Design review of the part built by this model. Coordinates are the model's own, in mm. Face numbers are marked on the shaded views. A direction names the side the tool comes from. Give positions to 0.01 mm unless a question says otherwise; leave off trailing zeros. Loops run counter-clockwise (first coordinate to the right, second up) from the corner with the lowest first, then second, coordinate; pieces in that order, holes last.
from build123d import *

# Parameters (mm, degrees)
SKETCH1_W           = 36
SKETCH1_H           = 36
BOSS_EXTRUDE1_DEPTH = 10
SKETCH2_W           = 25
SKETCH2_H           = 25
BOSS_EXTRUDE2_DEPTH = 2.5
SKETCH3_R           = 4
BOSS_EXTRUDE3_DEPTH = 12
SKETCH4_R           = 6.5
BOSS_EXTRUDE4_DEPTH = 5
SKETCH5_R           = 5
CUT_EXTRUDE1_DEPTH  = 3
FILLET1_R           = 4
FILLET2_R           = 4
SKETCH7_R           = 1.5
CUT_EXTRUDE2_DEPTH  = 5
SKETCH8_R           = 1.5
CUT_EXTRUDE3_DEPTH  = 5
FILLET3_R           = 1


with BuildPart() as part:
    # Sketch1 → Boss-Extrude1 (new body)
    with BuildSketch(Plane.XY):
        with Locations((18, 18)):
            Rectangle(SKETCH1_W, SKETCH1_H)
    extrude(amount=BOSS_EXTRUDE1_DEPTH)

    # Sketch2 → Boss-Extrude2 (add)
    with BuildSketch(Plane.XY.offset(10)):
        with Locations((18, 18)):
            Rectangle(SKETCH2_W, SKETCH2_H)
    extrude(amount=BOSS_EXTRUDE2_DEPTH)

    # Sketch3 → Boss-Extrude3 (add)
    with BuildSketch(Plane.XY.offset(12.5)):
        with Locations((18, 18)):
            Circle(SKETCH3_R)
    extrude(amount=BOSS_EXTRUDE3_DEPTH)

    # Sketch4 → Boss-Extrude4 (add)
    with BuildSketch(Plane.XY.offset(24.5)):
        with Locations((18, 18)):
            Circle(SKETCH4_R)
    extrude(amount=BOSS_EXTRUDE4_DEPTH)

    # Sketch5 → Cut-Extrude1 (cut)
    with BuildSketch(Plane.XY.offset(29.5)):
        with Locations((18, 18)):
            Circle(SKETCH5_R)
    extrude(amount=-CUT_EXTRUDE1_DEPTH, mode=Mode.SUBTRACT)

    # Sketch6 → Revolve4 (revolve)
    with BuildSketch(Plane.XY.offset(26.5)):
        with BuildLine():
            Line((18, 22), (18, 14))
            ThreePointArc((18, 14), (22, 18), (18, 22))
        make_face()
    revolve(axis=Axis((18, 22, 26.5), (0, -1, 0)))

    # Fillet1
    fillet1_edges = [part.edges().sort_by_distance(p)[0] for p in [
        (30.5, 5.5, 11.25),
        (30.5, 30.5, 11.25),
        (5.5, 30.5, 11.25),
        (5.5, 5.5, 11.25),
    ]]
    fillet(fillet1_edges, radius=FILLET1_R)

    # Fillet2
    fillet2_edges = [part.edges().sort_by_distance(p)[0] for p in [
        (0, 36, 5),
        (36, 36, 5),
        (36, 0, 5),
        (0, 0, 5),
    ]]
    fillet(fillet2_edges, radius=FILLET2_R)

    # Sketch7 → Cut-Extrude2 (cut)
    with BuildSketch(Plane(origin=(36, 0, 0), x_dir=(0, 0, -1), z_dir=(1, 0, 0))):
        with Locations((-5, 18)):
            Circle(SKETCH7_R)
    extrude(amount=-CUT_EXTRUDE2_DEPTH, mode=Mode.SUBTRACT)

    # Sketch8 → Cut-Extrude3 (cut)
    with BuildSketch(Plane.ZY):
        with Locations((5, 18)):
            Circle(SKETCH8_R)
    extrude(amount=-CUT_EXTRUDE3_DEPTH, mode=Mode.SUBTRACT)

    # Fillet3
    fillet3_edges = [part.edges().sort_by_distance(p)[0] for p in [
        (13, 18, 29.5),
    ]]
    fillet(fillet3_edges, radius=FILLET3_R)


solid = part.part
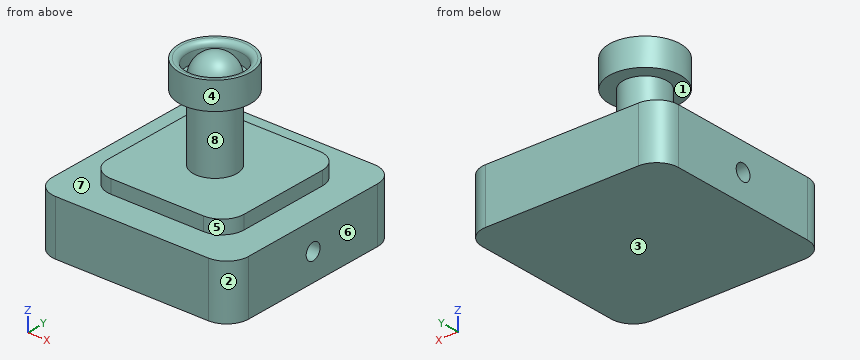
Q1. Draft analysis for pull direction Z (two halves, no side actions). For the marked faces 6, 7 and 8, state which applies: pulls with the +Z half, pulls with the -Z half, needs draft (parallel to the pull), parting line crosses it, or undercut.
Results:
face 6: needs draft
face 7: pulls with the +Z half
face 8: undercut
Q2. Wall thickness on line 1 (Y direction, x = 32, z = 5); line 2 (Z direction, x = 14, y = 23); line 3 (Y direction, x = 18, z = 27.8): over which ranges is each line inside the solid? List them lowest first.
Results:
line 1: y = 0 to 16.5, 19.5 to 36
line 2: z = 0 to 12.5, 24.5 to 29.5
line 3: y = 11.5 to 13, 14.22 to 21.78, 23 to 24.5
Q3. Take a section at B-B (x = 18). Give the boundary of the cut face in (y, z), plus the area to 3 significant figures.
Results:
outline: (0, 0) - (36, 0) - (36, 10) - (30.5, 10) - (30.5, 12.5) - (22, 12.5) - (22, 24.5) - (24.5, 24.5) - (24.5, 29.5) - (24, 29.5) arc R1 ccw to (23, 28.5) - (23, 26.5) - (22, 26.5) arc R4 ccw to (14, 26.5) - (13, 26.5) - (13, 28.5) arc R1 ccw to (12, 29.5) - (11.5, 29.5) - (11.5, 24.5) - (14, 24.5) - (14, 12.5) - (5.5, 12.5) - (5.5, 10) - (0, 10) - close
area: 578 mm2
Q4. Take a section at D-D (z = 22). Give the boundary of the cut face in (x, y).
Results:
outline: circle Ø8 at (18, 18)
Q5. Insertion check: pin 1 (0.9 mm diameter, centred on y = 17.5, z = 4.5, fed in from +X); pin 2 (6 mm diameter, centred on y = 27, z = 11.5, fed in from -X); pin 3 (1.2 mm diameter, centred on y = 22, z = 11.5, fed in from -X); pin 4 (0.8 mm diameter, centred on x = 15, z = 11.5, fed in from -Y). Each pin has a flat end and moves straight along its axis. Give the tip position at first contact, or say it passes through.
Results:
pin 1: stops at x = 31
pin 2: stops at x = 0
pin 3: stops at x = 5.5
pin 4: stops at y = 5.5
Q6. Take a section at A-A (z = 5). Give the boundary of the cut face in (x, y).
Results:
outline: (0, 4) arc R4 ccw to (4, 0) - (32, 0) arc R4 ccw to (36, 4) - (36, 16.5) - (31, 16.5) - (31, 19.5) - (36, 19.5) - (36, 32) arc R4 ccw to (32, 36) - (4, 36) arc R4 ccw to (0, 32) - (0, 19.5) - (5, 19.5) - (5, 16.5) - (0, 16.5) - close
Q7. Tool access review of the marked faces 1, 2, 3, 4 and 5: name each direction out of +Z, -Z, +X, -X, +Y, -Y from which nothing blocks a thin tool from reaching the whole face with its end or side.
Results:
face 1: none
face 2: +Z, -Z, +X, -Y
face 3: -Z, +X, -X, +Y, -Y
face 4: +Z
face 5: +Z, +X, -Y
